from build123d import *

# Parameters (mm, degrees)
SKETCH1_R           = 10
BOSS_EXTRUDE1_DEPTH = 15
SKETCH2_R           = 7.55
BOSS_EXTRUDE2_DEPTH = 15
FILLET1_R           = 0.5


with BuildPart() as part:
    # Sketch1 → Boss-Extrude1 (new body)
    with BuildSketch(Plane(origin=(0, 0, 0), x_dir=(1, 0, 0), z_dir=(0, 1, 0))):
        with Locations(Location((0, 0, 0), (0, 0, 270))):
            Circle(SKETCH1_R)
    extrude(amount=BOSS_EXTRUDE1_DEPTH)

    # Sketch2 → Boss-Extrude2 (add)
    with BuildSketch(Plane(origin=(0, 15, 0), x_dir=(1, 0, 0), z_dir=(0, 1, 0))):
        with Locations(Location((0, 0, 0), (0, 0, 270))):
            Circle(SKETCH2_R)
    extrude(amount=BOSS_EXTRUDE2_DEPTH)

    # Fillet1
    fillet1_edges = [part.edges().sort_by_distance(p)[0] for p in [
        (0, 0, -10),
        (0, 15, -10),
        (0, 15, -7.55),
        (0, 30, -7.55),
    ]]
    fillet(fillet1_edges, radius=FILLET1_R)


solid = part.part
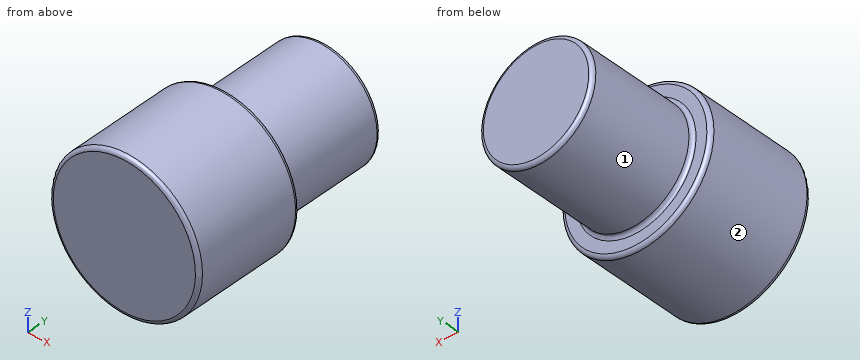
Build history of the part. All positions in model axes, mm. Face numbers are marked on the shaded views. A direction names the side the tool comes from. Round coordinates to 2 decimals unless told otherwise and drop trailing zeros. Write each loop counter-clockwise with the first axis right and the second up, starting at its lowest first coordinate (ties: lowest second). Pieces come first, ordered by that corner, then holes. Notation, with made-up numbers: M 55.25,50.5 L 68.25,50.5 A20 cw 68.25,89.5 Z; hole C -14,23.25 d7. An arc over 180 degrees is marked long. Answer as a JSON object with one key per item and string values. Group by question number.
(1) Cut at B-B (z = 0). Give the cut face in (x, y).
(2) Flat gauge pins, fed straight in: pin 1 (8 mm diameter, centred on x = -6, y = 19.5, fed in from +Z); pin 2 (2 mm diameter, centred on x = -4, y = 18, fed in from +Z); pin 3 (3 mm diameter, centred on y = 6.5, z = 5.5, fed in from -X). Where does each tip first touch, or does it go through?
(3) Drill centre lines: L1, parallel to Y at x = -2.5, z = 9.25; L2, parallel to X at y = 4.5, z = -7.75; L3, parallel to X at y = 4, z = -2.75. Where is each one in solid material? Low to high.
(4) Cut at C-C (y = 11.5). Give the cut face in (x, z), and give its area (3 significant figures).
(5) Cut at A-A (x = 0). Give the cut face in (y, z).
(6) Which spindle directions (+Z, -Z, +X, -X, +Y, -Y) get a long thin tool onto all of the face, cutting with end or side? Do the marked faces 1 and 2. Say none if no direction does.
(7) Cut at D-D (y = 19.75). Give the cut face in (x, z), and give its area (3 significant figures).
Responses:
{
 "1": {"outline": "M -10,0.5 A0.5 ccw -9.5,0 L 9.5,0 A0.5 ccw 10,0.5 L 10,14.5 A0.5 ccw 9.5,15 L 8.05,15 A0.5 cw 7.55,15.5 L 7.55,29.5 A0.5 ccw 7.05,30 L -7.05,30 A0.5 ccw -7.55,29.5 L -7.55,15.5 A0.5 cw -8.05,15 L -9.5,15 A0.5 ccw -10,14.5 Z"},
 "2": {"pin 1": "stops at z = 7.28", "pin 2": "stops at z = 6.93", "pin 3": "stops at x = -9.17"},
 "3": {"L1": "y = 0.01 to 14.99", "L2": "x = -6.32 to 6.32", "L3": "x = -9.61 to 9.61"},
 "4": {"outline": "C 0,0 d20", "area": "314 mm2"},
 "5": {"outline": "M 0,-9.5 A0.5 ccw 0.5,-10 L 14.5,-10 A0.5 ccw 15,-9.5 L 15,-8.05 A0.5 cw 15.5,-7.55 L 29.5,-7.55 A0.5 ccw 30,-7.05 L 30,7.05 A0.5 ccw 29.5,7.55 L 15.5,7.55 A0.5 cw 15,8.05 L 15,9.5 A0.5 ccw 14.5,10 L 0.5,10 A0.5 ccw 0,9.5 Z"},
 "6": {"face 1": "+Y", "face 2": "+Y, -Y"},
 "7": {"outline": "C 0,0 d15.1", "area": "179 mm2"}
}
